The figure shows three views and two pictorial views of one solid part (mm, origin at its lowest corner). Answer the questions. A direction names the side the tool comes from. Coordinates: 2 decimals unless noted, no trailing zeros. Loops run counter-clockwise (first coordinate to the right, second up) from the corner with the lowest first, then second, coordinate; pieces in that order, holes last. Notation, with made-up numbers: M 28.25,-5.75 L 40.25,-5.75 A20 ccw 40.25,3.25 Z; hole C -17.75,42 d10. An arc over 180 degrees is marked long. Answer in a Markdown table with one row per item. Add a question column.
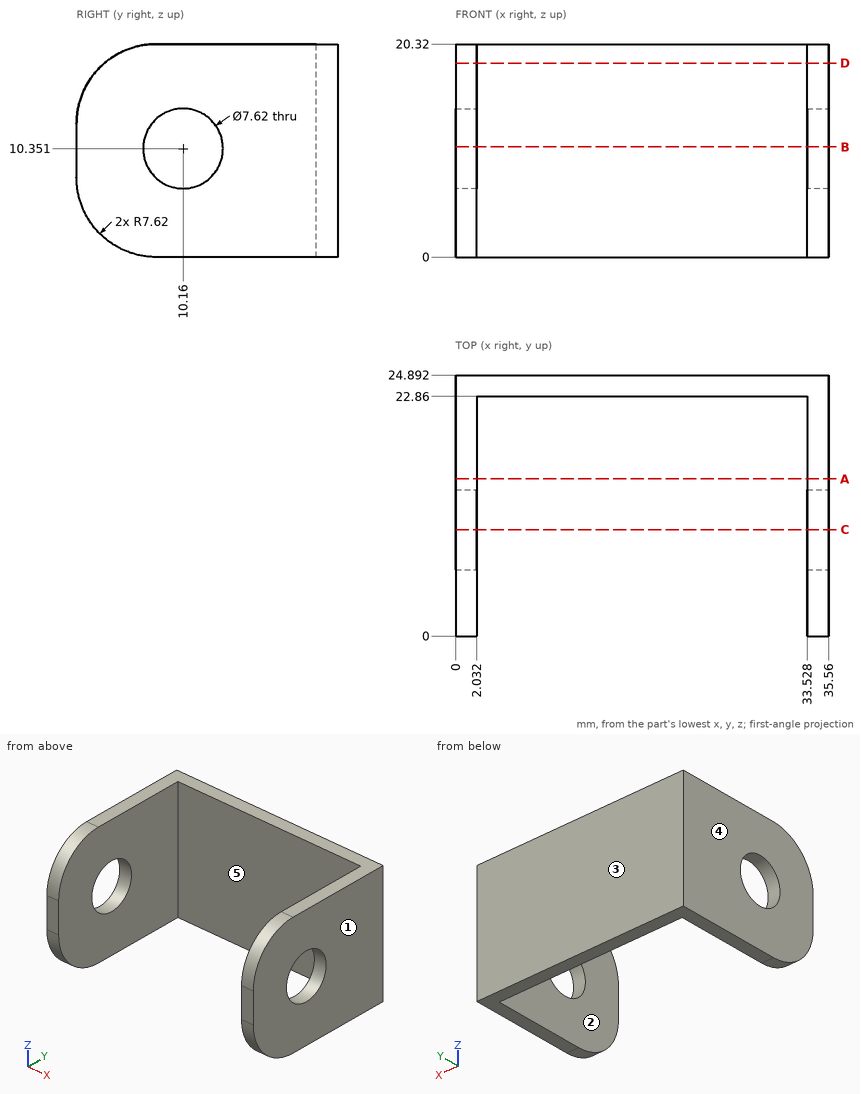
(1) A cutting plane is placed at A-A (y = 15). Give the vertices of the cut face in (x, z).
(2) A cutting plane is placed at C-C (y = 10.16). Give the vertices of the cut face in (x, z).
(3) For the marked faces 1 and 2, determine the directions among +Z, -Z, +X, -X, +Y, -Y from which every point of the face is accessible in a straight line to the end or side of a thin tool.
(4) A cutting plane is placed at B-B (z = 10.5). Give the vertices of the cut face in (x, y), plus the area to 3 significant figures.
(5) The mould has two halves that part along X. Classify the marked faces 3, 4 and 5: released by +X, released by -X, zero draft, split by the parting line, or undercut.
(6) A cutting plane is placed at D-D (z = 18.5). Give the vertices of the cut face in (x, y), plus the area to 3 significant figures.
(7) Straight lines are drawn through the part: line 1 (X direction, y = 14.5, z = 15); line 2 (Y direction, x = 31, z = 3.75). For each, find the intervals that lie inside material, in ascending order.
Solved:
| question | item | result |
|---|---|---|
| 1 | outline | M 0,0 L 2.03,0 L 2.03,20.32 L 0,20.32 Z; M 33.53,0 L 35.56,0 L 35.56,20.32 L 33.53,20.32 Z |
| 2 | outline | M 0,0 L 2.03,0 L 2.03,6.54 L 0,6.54 Z; M 0,14.16 L 2.03,14.16 L 2.03,20.32 L 0,20.32 Z; M 33.53,0 L 35.56,0 L 35.56,6.54 L 33.53,6.54 Z; M 33.53,14.16 L 35.56,14.16 L 35.56,20.32 L 33.53,20.32 Z |
| 3 | face 1 | +Z, -Z, +X, +Y, -Y |
| 3 | face 2 | +Z, -Z, -Y |
| 4 | outline | M 0,0 L 2.03,0 L 2.03,6.35 L 0,6.35 Z; M 0,13.97 L 2.03,13.97 L 2.03,22.86 L 33.53,22.86 L 33.53,13.97 L 35.56,13.97 L 35.56,24.89 L 0,24.89 Z; M 33.53,0 L 35.56,0 L 35.56,6.35 L 33.53,6.35 Z |
| 4 | area | 134 mm² |
| 5 | face 3 | zero draft |
| 5 | face 4 | released by -X |
| 5 | face 5 | undercut |
| 6 | outline | M 0,2.68 L 2.03,2.68 L 2.03,22.86 L 33.53,22.86 L 33.53,2.68 L 35.56,2.68 L 35.56,24.89 L 0,24.89 Z |
| 6 | area | 154 mm² |
| 7 | line 1 | x = 0 to 2.03, 33.53 to 35.56 |
| 7 | line 2 | y = 22.86 to 24.89 |
